Read the model definition and answer for the solid it produces. Units are mm, in the model's axes. Face numbers are marked on the shaded views. Coordinates: 2 decimals unless noted, no trailing zeros. Order: outer loops, then holes, each group sorted by start corner. A loop starts at its lowest first (then second) coordinate and runs counter-clockwise, first axis right, second up. Notation, with made-up numbers: M -19,13.5 L 20,13.5 A13 cw 20,34.5 Z; hole C 61,64.5 d1. An arc over 180 degrees is marked long. Use a Markdown table: item, result. Add a question column.
1) Find section D-D on z = -16.5. Write down the section's boundary in (x, y) (3 decimals), plus the area to 3 significant figures.
2) This flat-tipped pin is pushed along its axis until it touches: pin 1 Ø1 at (y, z) = (-15.5, -25) entering from +X. Where does it stop, or does it pass through?
3) Find the intervals of material crossed by probe 1 along Z at (x, y) = (21, 0) (3 decimals); probe 2 along Y at (x, z) = (14.5, -6) (3 decimals); probe 3 along X at (y, z) = (-20, -10), in increasing order. Write a range as [from, to].
4) Find section C-C on x = 21.5. Write down the section's boundary in (y, z) (3 decimals), plus the area to 3 significant figures.
5) Find section B-B on z = -26.5. Write down the section's boundary in (x, y) (3 decimals).
6) The mould has two halves that part along Y. Classify the marked faces 1, 2 and 3: released by +Y, released by -Y, zero draft, split by the parting line, or undercut.
7) Find section A-A on y = 0. Write down the section's boundary in (x, z) (3 decimals).
from build123d import *

# Parameters (mm, degrees)
F0_R     = 19.05
F1_DEPTH = 12.7
F0_W     = 44.45
F0_H     = 82.55
F2_DEPTH = 31.75
F3_R     = 2.54


with BuildPart() as f1:
    # F0 (on Right) → F1 (new body)
    with BuildSketch(Plane.YZ):
        with Locations((0, -18.576264)):
            Circle(F0_R)
    extrude(amount=F1_DEPTH)

    # F0 (on Right) → F2 (join)
    with BuildSketch(Plane.YZ):
        Rectangle(F0_W, F0_H)
        with Locations((0, -18.576264)):
            Circle(F0_R, mode=Mode.SUBTRACT)
    extrude(amount=F2_DEPTH)

    # F3
    f3_edges = [f1.edges().sort_by_distance(p)[0] for p in [
        (15.875, -22.225, -41.275),
        (15.875, 22.225, -41.275),
        (0, 0, -41.275),
        (31.75, 0, -41.275),
        (31.75, 22.225, 0),
        (0, 22.225, 0),
        (0, -22.225, 0),
        (31.75, -22.225, 0),
    ]]
    fillet(f3_edges, radius=F3_R)


solid = f1.part
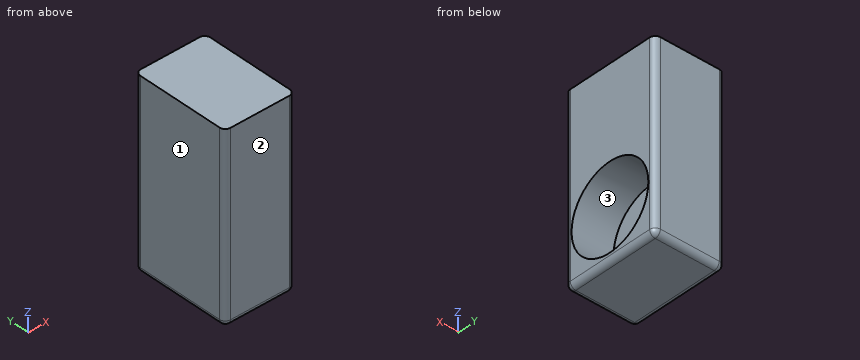
Check result:
| question | item | result |
|---|---|---|
| 1 | outline | M 0,-19.685 A2.54 ccw 2.54,-22.225 L 29.21,-22.225 A2.54 ccw 31.75,-19.685 L 31.75,-18.937 L 12.7,-18.937 L 12.7,18.937 L 31.75,18.937 L 31.75,19.685 A2.54 ccw 29.21,22.225 L 2.54,22.225 A2.54 ccw 0,19.685 Z |
| 1 | area | 684 mm2 |
| 2 | pin 1 | stops at x = 12.7 |
| 3 | probe 1 | z = [-41.275, -37.626], [0.474, 41.275] |
| 3 | probe 2 | y = [-22.225, -14.309], [14.309, 22.225] |
| 3 | probe 3 | x = [0.02, 31.73] |
| 4 | outline | M -22.225,-38.735 A2.54 ccw -19.685,-41.275 L 19.685,-41.275 A2.54 ccw 22.225,-38.735 L 22.225,41.275 L -22.225,41.275 Z; hole C 0,-18.576 d38.1 |
| 4 | area | 2,530 mm2 |
| 5 | outline | M 0,-19.685 A2.54 ccw 2.54,-22.225 L 29.21,-22.225 A2.54 ccw 31.75,-19.685 L 31.75,-17.324 L 12.7,-17.324 L 12.7,17.324 L 31.75,17.324 L 31.75,19.685 A2.54 ccw 29.21,22.225 L 2.54,22.225 A2.54 ccw 0,19.685 Z |
| 6 | face 1 | zero draft |
| 6 | face 2 | released by -Y |
| 6 | face 3 | undercut |
| 7 | outline | M 0,-38.735 A2.54 ccw 2.54,-41.275 L 29.21,-41.275 A2.54 ccw 31.75,-38.735 L 31.75,-37.626 L 12.7,-37.626 L 12.7,0.474 L 31.75,0.474 L 31.75,41.275 L 0,41.275 Z |
